Autodesk Inventor part; units mm, degrees
ref_plane "YZ Plane" through (0, 0, 0) normal (1, 0, 0) x (0, 1, 0)
ref_plane "XZ Plane" through (0, 0, 0) normal (0, 1, 0) x (-1, 0, 0)
ref_plane "XY Plane" through (0, 0, 0) normal (0, 0, 1) x (1, 0, 0)
sketch "Sketch1" plane through (0, 0, 0) normal (0, 0, 1) x (1, 0, 0)
  line L0 (0, 0) -> (12.7, 0)
  line L1 (12.7, 0) -> (12.7, 22.86)
  line L2 (0, 0) -> (0, 35.56)
  line L3 (0, 35.56) -> (139.7, 35.56)
  line L4 (139.7, 35.56) -> (139.7, 0.56)
  line L5 (139.7, 0.56) -> (127, 0.56)
  line L6 (127, 0.56) -> (127, 22.86)
  line L7 (127, 22.86) -> (12.7, 22.86)
  line L8 (6.35, 28.6931) -> (133.35, 28.6931) construction
  line L9 (6.35, 28.6931) -> (6.35, 0) construction
  line L10 (133.35, 28.6931) -> (133.35, 0) construction
  dimension "d0" = 12.7
  dimension "d2" = 35.56
  dimension "d4" = 12.7
  dimension "d28" = 12.7
  dimension "d29" = 127
extrude "Extrusion1" add sketch "Sketch1" along normal blind 12.7
hole "Hole1" at (6.35, 0, 6.35) direction (0, 1, 0) diameter 4.3434 depth 25
hole "Hole2" at (133.35, 0.56, 6.35) direction (0, 1, 0) diameter 4.3434 depth 25
properties part number "BarHandle5in" material "Stainless Steel"
Could you check a few things on this model? Use its own coordinates, in mm. A direction names the side the tool comes from. Round coordinates to 2 decimals unless told otherwise and drop trailing zeros. Loops run counter-clockwise (first coordinate to the right, second up) from the corner with the lowest first, then second, coordinate; pieces in that order, holes last. Notation, with made-up numbers: (84.5, 74) - (140.5, 74) arc R31 ccw to (140.5, 105) - close; hole circle Ø1 at (44.25, -33). An arc over 180 degrees is marked (long way). Answer in a Markdown table with one row per item. Add a question column.
(1) If we mould it in two halves opening along Z, with no side actions, what happens to faces 1 (the face through (127, 12, 6)), 2 (the face through (6, 25, 6)), 3 (the face through (69, 26, 12.7)), 4 (the face through (69, 26, 0))? For each: pulls with the +Z half, pulls with the -Z half, needs draft (parallel to the pull), parting line crosses it, or undercut.
(2) If we section it at D-D (x = 86.5): Please give me the cut outline in (y, z), plus the area to 3 significant figures.
(3) If we section it at C-C (z = 1.75): Please give me the cut outline in (x, y), plus the area to 3 significant figures.
(4) If we section it at B-B (x = 133.35): Please give me the cut outline in (y, z).
(5) I'm going to push flat-ended pins straight in: pin 1 (3.5 mm diameter, centred on x = 6, z = 5.5, fed in from -Y); pin 2 (2 mm diameter, centred on x = 132.5, z = 5.5, fed in from -Y); pin 3 (5 mm diameter, centred on x = 90.5, z = 10, fed in from -Y). Where does each tip first touch, or does it pass through?
(6) For faces 5 (the face through (135.47, 13.24, 6.82)), 6 (the face through (131, 0.56, 6)), 7 (the face through (69, 35.56, 6)), 8 (the face through (71, 22.86, 6)), which set-ups out of +Z, -Z, +X, -X, +Y, -Y let a thin tool reach every point of the face, with its end or its side?
(7) I need wall thicknesses on line 1 along X through (y, z) = (6.25, 6.35); line 2 along X through (y, z) = (5, 12.25); line 3 along Z through (x, y) = (6.35, 7). Which ranges of each line are inside material? Lowest first, please.
(8) If we section it at A-A (y = 6): Please give me the cut outline in (x, z), plus the area to 3 significant figures.
Model answer:
| question | item | result |
|---|---|---|
| 1 | face 1 | needs draft |
| 1 | face 2 | undercut |
| 1 | face 3 | pulls with the +Z half |
| 1 | face 4 | pulls with the -Z half |
| 2 | outline | (22.86, 0) - (35.56, 0) - (35.56, 12.7) - (22.86, 12.7) - close |
| 2 | area | 161 mm² |
| 3 | outline | (0, 0) - (12.7, 0) - (12.7, 22.86) - (127, 22.86) - (127, 0.56) - (139.7, 0.56) - (139.7, 35.56) - (0, 35.56) - close |
| 3 | area | 2,350 mm² |
| 4 | outline | (0.56, 0) - (35.56, 0) - (35.56, 12.7) - (0.56, 12.7) - (0.56, 8.52) - (25.56, 8.52) - (25.56, 4.18) - (0.56, 4.18) - close |
| 5 | pin 1 | stops at y = 0 |
| 5 | pin 2 | stops at y = 0.56 |
| 5 | pin 3 | stops at y = 22.86 |
| 6 | face 5 | -Y |
| 6 | face 6 | +Z, -Z, +X, -Y |
| 6 | face 7 | +Z, -Z, +X, -X, +Y |
| 6 | face 8 | +Z, -Z, -Y |
| 7 | line 1 | x = 0 to 4.18, 8.52 to 12.7, 127 to 131.18, 135.52 to 139.7 |
| 7 | line 2 | x = 0 to 12.7, 127 to 139.7 |
| 7 | line 3 | z = 0 to 4.18, 8.52 to 12.7 |
| 8 | outline | (0, 0) - (12.7, 0) - (12.7, 12.7) - (0, 12.7) - close; (127, 0) - (139.7, 0) - (139.7, 12.7) - (127, 12.7) - close; hole circle Ø4.34 at (6.35, 6.35); hole circle Ø4.34 at (133.35, 6.35) |
| 8 | area | 293 mm² |
